For this review, use the dimensioned drawing (mm, ordinates from the lowest corner) and the shaded views. A direction names the side the tool comes from. Coordinates: 2 decimals unless noted, no trailing zeros. Write each loop counter-clockwise with the first axis right and the second up, starting at its lowest first coordinate (ties: lowest second). Pieces come first, ordered by that corner, then holes.
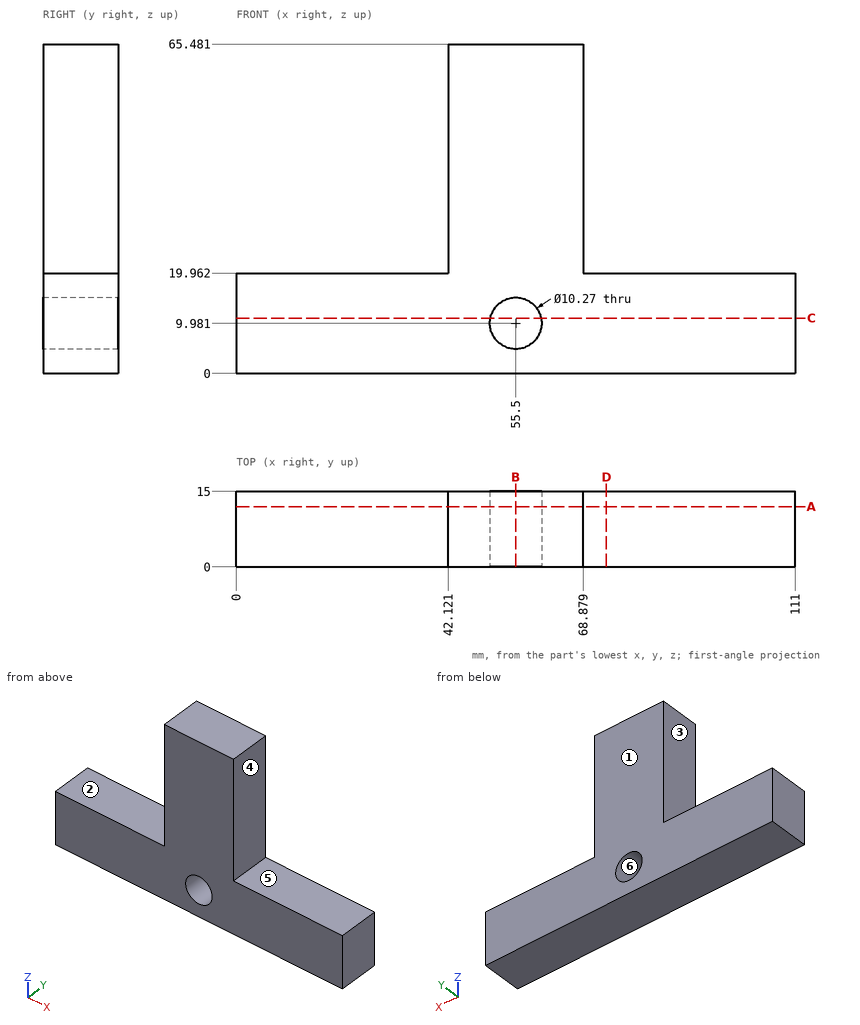
Item 1: Take a section at D-D, the plane x = 73.5. Write out the cut boundary in (y, z), plus the area to 3 significant figures.
Solved:
outline: (0, 0) - (15, 0) - (15, 19.96) - (0, 19.96) - close
area: 299 mm2
Item 2: Take a section at A-A, the plane y = 12. Write out the cut boundary in (x, z) (1 decimal), plus the area to 3 significant figures.
Solved:
outline: (0, 0) - (111, 0) - (111, 20) - (68.9, 20) - (68.9, 65.5) - (42.1, 65.5) - (42.1, 20) - (0, 20) - close; hole circle Ø10.3 at (55.5, 10)
area: 3,350 mm2
Item 3: Machinability: for the marked faces 1 and 2, which of the approach directions +Z, -Z, +X, -X, +Y, -Y give a long, thin tool a straight path to every point of the face, cutting with its end or side? Answer none if there is none.
Solved:
face 1: +Z, -Z, +X, -X, +Y
face 2: +Z, -X, +Y, -Y
Item 4: Take a section at B-B, the plane x = 55.5. Write out the cut boundary in (y, z), plus the area to 3 significant figures.
Solved:
outline: (0, 0) - (15, 0) - (15, 4.85) - (0, 4.85) - close; (0, 15.12) - (15, 15.12) - (15, 65.48) - (0, 65.48) - close
area: 828 mm2
Item 5: For pin 1 (8 mm diameter, centred on y = 7.5, z = 54.5, fed in from -X); pin 2 (3 mm diameter, centred on x = 23.5, y = 9.5, fed in from +Z), all flat-tipped, find the tip position at first contact; note any pin that passes through.
Solved:
pin 1: stops at x = 42.12
pin 2: stops at z = 19.96
Item 6: Take a section at C-C, the plane z = 11. Write out the cut boundary in (x, y), plus the area to 3 significant figures.
Solved:
outline: (0, 0) - (50.47, 0) - (50.47, 15) - (0, 15) - close; (60.53, 0) - (111, 0) - (111, 15) - (60.53, 15) - close
area: 1,510 mm2
Item 7: To check wall thickness, follow line 1 along X through (y, z) = (1, 23); line 2 along Z through (x, y) = (12.5, 14.25); line 3 along X through (y, z) = (2, 9). State the ranges of each line that lie inside material, in increasing order.
Solved:
line 1: x = 42.12 to 68.88
line 2: z = 0 to 19.96
line 3: x = 0 to 50.46, 60.54 to 111
Item 8: Mouldability with a two-part tool opening along X and no side actions: class the marked faces 3, 4, 5 and 6 as pulls with the +X half, pulls with the -X half, needs draft (parallel to the pull), parting line crosses it, or undercut.
Solved:
face 3: pulls with the -X half
face 4: pulls with the +X half
face 5: needs draft
face 6: undercut
